from build123d import *

# Parameters (mm, degrees)
BOSS_EXTRUDE1_DEPTH = 15
SKETCH2_W           = 10.25
SKETCH2_H           = 10.25
CUT_EXTRUDE1_DEPTH  = 18
SKETCH3_W           = 10.25
SKETCH3_H           = 10.25
CUT_EXTRUDE2_DEPTH  = 17
CUT_EXTRUDE3_REACH  = 41.336
SKETCH4_W           = 8
SKETCH4_H           = 8
CUT_EXTRUDE4_REACH  = 34.317
SKETCH5_W           = 8
SKETCH5_H           = 8
FILLET1_R           = 6
FILLET2_R           = 3
BOSS_EXTRUDE2_DEPTH = 15


with BuildPart() as part:
    # Sketch1 → Boss-Extrude1 (new body)
    with BuildSketch(Plane(origin=(0, 0, 0), x_dir=(1, 0, 0), z_dir=(0, 1, 0))):
        Polygon((0, 0), (15.436230849, -4.13612559), (19.318516526, 10.352761804), (0, 15.529142706), (-3.882285677, 30.0180301), (-18.371173071, 26.135744424), (-10.606601718, -2.842030365), align=None)
    extrude(amount=BOSS_EXTRUDE1_DEPTH)

    # Sketch2 → Cut-Extrude1 (cut)
    with BuildSketch(Plane(origin=(15.436230849, 0, 4.13612559), x_dir=(0.2588190451025214, 0, -0.9659258262890681), z_dir=(0.9659258262890681, 0, 0.2588190451025214))):
        with Locations((7.5, 7.5)):
            Rectangle(SKETCH2_W, SKETCH2_H)
    extrude(amount=-CUT_EXTRUDE1_DEPTH, mode=Mode.SUBTRACT)

    # Sketch3 → Cut-Extrude2 (cut)
    with BuildSketch(Plane(origin=(-7.764571353, 0, -28.977774789), x_dir=(-0.9659258262890682, 0, 0.2588190451025212), z_dir=(-0.2588190451025212, 0, -0.9659258262890682))):
        with Locations((3.480762114, 7.5)):
            Rectangle(SKETCH3_W, SKETCH3_H)
    extrude(amount=-CUT_EXTRUDE2_DEPTH, mode=Mode.SUBTRACT)

    # Cut-Extrude3: up to this plane
    cut_extrude3_end = Plane(origin=(-11.677175467, 12.625, -10.329700609), z_dir=(-0.9659258262890682, 0, 0.2588190451025212))
    # Sketch4 → Cut-Extrude3 (cut, up to the surface)
    with BuildSketch(Plane(origin=(-1.950434024, 0, -0.522617222), x_dir=(0.25881904510252146, 0, -0.9659258262890681), z_dir=(0.9659258262890681, 0, 0.25881904510252146)), mode=Mode.PRIVATE) as cut_extrude3_sk1:
        with Locations((7.5, 7.5)):
            Rectangle(SKETCH4_W, SKETCH4_H)
    cut_extrude3_tool1 = split(extrude(cut_extrude3_sk1.sketch, amount=-CUT_EXTRUDE3_REACH, mode=Mode.PRIVATE), bisect_by=cut_extrude3_end, keep=Keep.BOTH, mode=Mode.PRIVATE)
    add(cut_extrude3_tool1.solids().sort_by_distance((-0.009291, 7.5, -7.767061))[0], mode=Mode.SUBTRACT)

    # Cut-Extrude4: up to this face of the body (flat: up to its plane)
    cut_extrude4_end = Plane(part.part.faces().sort_by_distance((-5.844526251, 7.5, -5.189502721))[0])
    # Sketch5 → Cut-Extrude4 (cut, up to the picked face)
    with BuildSketch(Plane(origin=(-3.364647586, 0, -12.557035742), x_dir=(-0.9659258262890682, 0, 0.25881904510252124), z_dir=(-0.25881904510252124, 0, -0.9659258262890682)), mode=Mode.PRIVATE) as cut_extrude4_sk1:
        with Locations((3.480762114, 7.5)):
            Rectangle(SKETCH5_W, SKETCH5_H)
    cut_extrude4_tool1 = split(extrude(cut_extrude4_sk1.sketch, amount=-CUT_EXTRUDE4_REACH, mode=Mode.PRIVATE), bisect_by=cut_extrude4_end, keep=Keep.BOTH, mode=Mode.PRIVATE)
    add(cut_extrude4_tool1.solids().sort_by(Axis((-6.726806, 7.5, -11.656148), (0.25881904510252124, 0, 0.9659258262890682)))[0], mode=Mode.SUBTRACT)

    # Fillet1
    fillet1_edges = [part.edges().sort_by_distance(p)[0] for p in [
        (-10.644485136, 7.5, -6.475647828),
    ]]
    fillet(fillet1_edges, radius=FILLET1_R)

    # Fillet2
    fillet2_edges = [part.edges().sort_by_distance(p)[0] for p in [
        (-11.609118038, 11.5, -10.075706826),
        (-0.915876519, 11.5, -12.151084448),
        (-0.915876519, 3.5, -12.151084448),
        (-11.609118038, 3.5, -10.075706826),
        (-4.171493644, 3.5, -4.741214984),
        (-9.988146338, 3.5, -7.131986626),
        (-4.171493644, 11.5, -4.741214984),
        (-9.988146338, 11.5, -7.131986626),
    ]]
    fillet(fillet2_edges, radius=FILLET2_R)

    # Sketch6 → Boss-Extrude2 (add)
    with BuildSketch(Plane(origin=(0, 15, 0), x_dir=(1, 0, 0), z_dir=(0, 1, 0))):
        Polygon((-10.606601718, -2.842030365), (-22.033626934, 0.219831814), (-16.730326075, 20.012020067), align=None)
    extrude(amount=-BOSS_EXTRUDE2_DEPTH)


solid = part.part
Check sheet for the modelled part. Datum: model origin and axes. Units: mm. A direction names the side the tool comes from. Give positions to 0.01 mm unless a question says otherwise; leave off trailing zeros. Loops run counter-clockwise (first coordinate to the right, second up) from the corner with the lowest first, then second, coordinate; pieces in that order, holes last. Notation, with made-up numbers: M 12.25,88.25 L 17.25,88.25 A8 cw 17.25,99.25 Z; hole C 53.25,73.25 d10. An arc over 180 degrees is marked long. Answer as a JSON object with one key per item and string values. Group by question number.
Q1. Material ranges on line 1 along Y through (x, z) = (-10.5, -19.5) (3 decimals); line 2 along Y through (x, z) = (-6.5, -10); line 3 along Z through (x, y) = (12, 3.5), recorded low to high. Write a range as [from, to].
Q2. Release check for a two-part mould opening along Z. For faces 4 (the cylindrical face through (-3.99, 4.4, -5.58)), 5 (the flat face through (-13.84, 7.43, -18.4)), 6 (the flat face through (19.076, 7.395, -9.446)), 7 (the flat face through (-1, 0, -9)) record: released by +Z, released by -Z, zero draft, split by the parting line, or undercut.
Q3. Access from +Z, -Z, +X, -X, +Y, -Y to the whole of each face (thin tool, end or side, straight path). Record for faces 1 (the flat face through (-4, 3.5, -10)), 2 (the cylindrical face through (-10.74, 10.64, -10.31)), 3 (the flat face through (-4.13, 7.49, -4.73)).
Q4. Cross-section at B-B on x = 13. Record the cut outline in (y, z) (3 decimals).
Q5. Go/stop test with flat-tipped pins: P1, Ø1, axis at x = -9, y = 5, coming from the -Z side; P2, Ø4, axis at y = 1.5, z = -24, coming from the -X side; P3, Ø5, axis at y = 10, z = -9.5, coming from the +X side. Record where each tip stops, or that it passes through.
Q6. Cross-section at D-D on x = 17.5. Record the cut outline in (y, z) (3 decimals), then the cut area to 3 significant figures.
Q7. Cross-section at C-C on z = -14. Record the cut outline in (x, y) (3 decimals).
Evaluation:
{
 "1": {"line 1": "y = [0, 2.375], [12.625, 15]", "line 2": "y = [0, 3.5], [11.5, 15]", "line 3": "z = [-12.31, -9.85], [0.76, 3.22]"},
 "2": {"face 4": "undercut", "face 5": "released by -Z", "face 6": "released by +Z", "face 7": "zero draft"},
 "3": {"face 1": "none", "face 2": "-Z", "face 3": "+X"},
 "4": {"outline": "M 0,-12.046 L 15,-12.046 L 15,3.483 L 0,3.483 Z; hole M 2.375,-9.587 L 12.625,-9.587 L 12.625,1.025 L 2.375,1.025 Z"},
 "5": {"P1": "stops at z = -7.41", "P2": "stops at x = -18.33", "P3": "stops at x = 19.32"},
 "6": {"outline": "M 0,-10.84 L 15,-10.84 L 15,-3.566 L 12.625,-3.566 L 12.625,-8.381 L 2.375,-8.381 L 2.375,-3.566 L 0,-3.566 Z", "area": "59.8 mm2"},
 "7": {"outline": "M -18.341,0 L 5.707,0 L 5.707,15 L -18.341,15 Z; hole M -12.661,2.375 L -2.049,2.375 L -2.049,12.625 L -12.661,12.625 Z"}
}
